Source: three-view drawing plus pictorial views. Frame: mm from the lowest corner of the part. A direction names the side the tool comes from. Coordinates: 2 decimals unless noted, no trailing zeros. Order: outer loops, then holes, each group sorted by start corner. A loop starts at its lowest first (then second) coordinate and runs counter-clockwise, first axis right, second up. Notation, with made-up numbers: M 18.25,1 L 57.25,1 A33 cw 57.25,34 Z; hole C -10.5,-26 d2. An arc over 180 degrees is marked long. Write item = value, one per line. Start each with the question number.
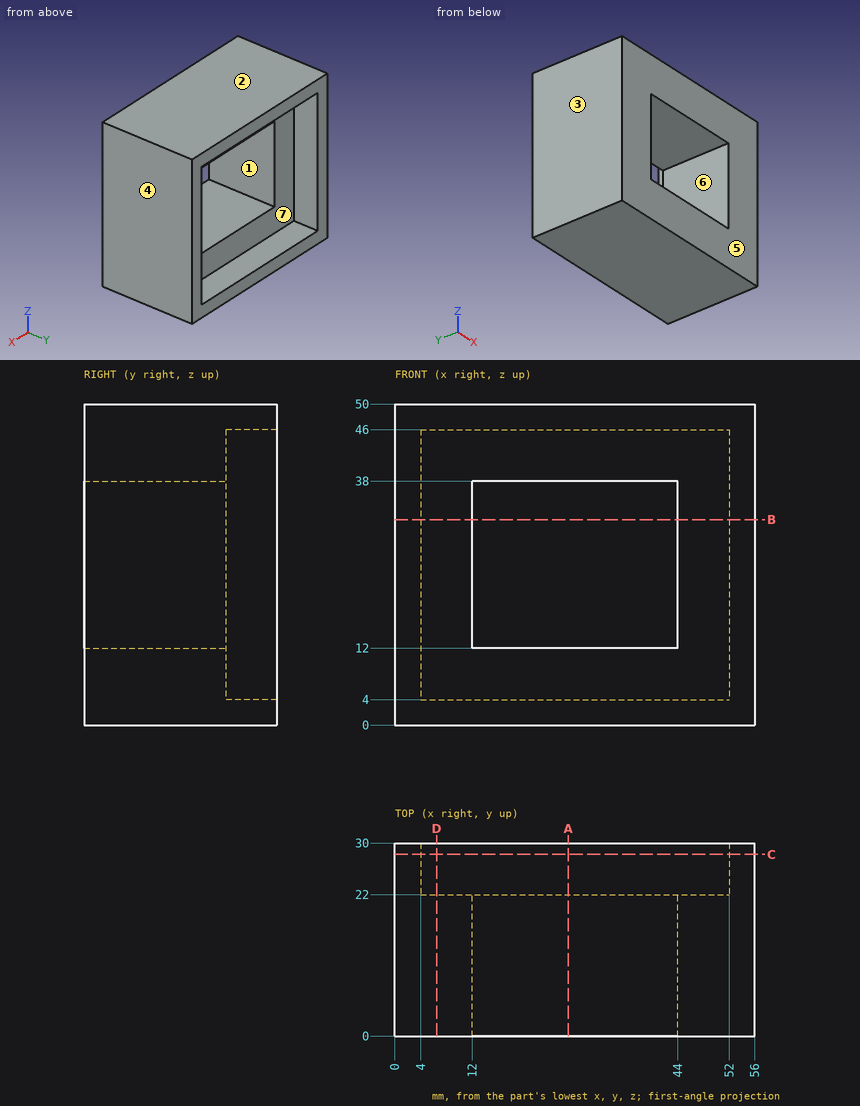
Item 1: Reachability of the marked faces 5, 6 and 7 from +Z, -Z, +X, -X, +Y, -Y: full face, straight path, thin tool, end or side. Return the list, or none.
Item 2: Section query A-A on x = 27. Output: boundary loops of the cut face in (y, z).
Item 3: Section query D-D on x = 6.5. Output: boundary loops of the cut face in (y, z).
Item 4: Section query C-C on y = 28.25. Output: boundary loops of the cut face in (x, z), and give its area (3 significant figures).
Item 5: Material intervals for probe 1 along X at (y, z) = (8.25, 16); probe 2 along Z at (x, y) = (38.5, 2.5); probe 3 along X at (y, z) = (26.5, 43.5), sorted ascending. Write a range as [from, to].
Item 6: Draft query along X for the marked faces 1, 2, 3 and 4. Return one class per face: pulls with the +X half, pulls with the -X half, needs draft (parallel to the pull), parting line crosses it, or undercut.
Item 7: Section query B-B on z = 32. Output: boundary loops of the cut face in (x, y).
Ans:
q1.face_5 = +Z, -Z, +X, -X, -Y
q1.face_6 = +Y, -Y
q1.face_7 = +Y
q2.outline = M 0,0 L 30,0 L 30,4 L 22,4 L 22,12 L 0,12 Z; M 0,38 L 22,38 L 22,46 L 30,46 L 30,50 L 0,50 Z
q3.outline = M 0,0 L 30,0 L 30,4 L 22,4 L 22,46 L 30,46 L 30,50 L 0,50 Z
q4.outline = M 0,0 L 56,0 L 56,50 L 0,50 Z; hole M 4,4 L 52,4 L 52,46 L 4,46 Z
q4.area = 784 mm^2
q5.probe_1 = [0, 12], [44, 56]
q5.probe_2 = [0, 12], [38, 50]
q5.probe_3 = [0, 4], [52, 56]
q6.face_1 = undercut
q6.face_2 = needs draft
q6.face_3 = pulls with the -X half
q6.face_4 = pulls with the +X half
q7.outline = M 0,0 L 12,0 L 12,22 L 4,22 L 4,30 L 0,30 Z; M 44,0 L 56,0 L 56,30 L 52,30 L 52,22 L 44,22 Z
